The model under review builds one solid part; all positions refer to its coordinate system, in mm. Face numbers are marked on the shaded views. A direction names the side the tool comes from. Coordinates: 2 decimals unless noted, no trailing zeros. Loops run counter-clockwise (first coordinate to the right, second up) from the corner with the lowest first, then second, coordinate; pieces in that order, holes last. Notation, with made-up numbers: M -38,5.25 L 2,5.25 A23 ccw 2,38.25 Z; hole C -34,-21.5 d4. An arc over 180 degrees is marked long. Return JSON: item names as keys, results as strings.
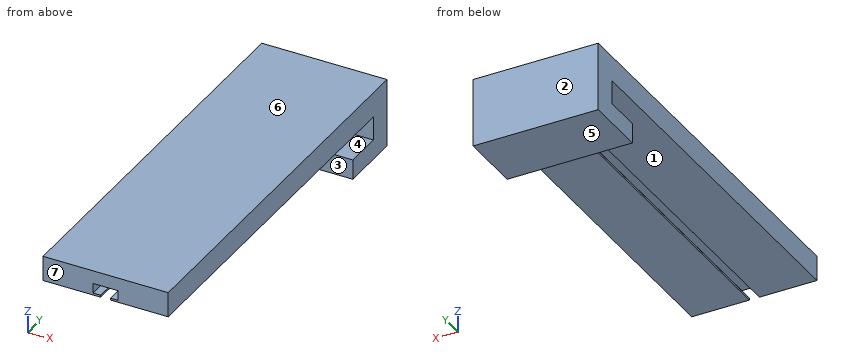
```python
from build123d import *

# Parameters (mm, degrees)
F0_W     = 15.875
F0_H     = 50.8
F1_DEPTH = 3.175
F2_W     = 15.875
F2_H     = 3.175
F3_DEPTH = 5.55625
F4_W     = 15.875
F4_H     = 2.54
F5_DEPTH = 4.7625
F6_W     = 1.27
F6_H     = 0.2512368413
F7_DEPTH = 38.1


with BuildPart() as f1:
    # F0 (on Top) → F1 (new body)
    with BuildSketch(Plane.XY):
        Rectangle(F0_W, F0_H)
    extrude(amount=F1_DEPTH)

    # F2 (on face) → F3 (join)
    with BuildSketch(Plane(origin=(0, 0, 0), x_dir=(1, 0, 0), z_dir=(0, 0, -1))):
        with Locations((0, -23.8125)):
            Rectangle(F2_W, F2_H)
    extrude(amount=F3_DEPTH)

    # F4 (on face) → F5 (join)
    with BuildSketch(Plane.XZ.offset(-22.225)):
        with Locations((0, -4.28625)):
            Rectangle(F4_W, F4_H)
    extrude(amount=F5_DEPTH)

    # F6 (on face) → F7 (cut)
    with BuildSketch(Plane.XZ.offset(25.4)):
        Polygon((0.635, 0.2512368413), (1.5875, 0.2512368413), (1.5875, 1.5212368413), (-1.5875, 1.5212368413), (-1.5875, 0.2512368413), (-0.635, 0.2512368413), align=None)
        with Locations((0, 0.1256184207)):
            Rectangle(F6_W, F6_H)
    extrude(amount=-F7_DEPTH, mode=Mode.SUBTRACT)


solid = f1.part
```
1. Add section C-C on z = -1.75. Give the boundary of the cut face in (x, y) (1 decimal), plus the area to 3 significant figures.
Check values:
{"outline": "M -7.9,22.2 L 7.9,22.2 L 7.9,25.4 L -7.9,25.4 Z", "area": "50.4 mm²"}
2. Add section B-B on x = -3.25. Give the boundary of the cut face in (y, z) (1 decimal).
Check values:
{"outline": "M -25.4,0 L 22.2,0 L 22.2,-3 L 17.5,-3 L 17.5,-5.6 L 25.4,-5.6 L 25.4,3.2 L -25.4,3.2 Z"}
3. To check wall thickness, follow line 1 (X direction, y = -3, z = 1); line 2 (Z direction, x = -6.25, y = 5) (3 decimals); line 3 (Y direction, x = 4, z = -3.5). State the ranges of each line that lie inside material, in increasing order.
Check values:
{"line 1": "-7.94 to -1.59, 1.59 to 7.94", "line 2": "0 to 3.175", "line 3": "17.46 to 25.4"}
4. Insertion check: pin 1 Ø1 at (x, y) = (0.5, -12.5) entering from -Z; pin 2 Ø1.5 at (x, z) = (0.5, -1) entering from -Y (3 decimals); pin 3 Ø0.5 at (x, z) = (0.5, 1) entering from -Y. Each pin has a flat end and moves straight along its axis. Give the tip position at first contact, or say it passes through.
Check values:
{"pin 1": "z = 0", "pin 2": "y = 22.225", "pin 3": "y = 12.7"}
5. Machinability: for the marked faces 1, 2 and 3, which of the approach directions +Z, -Z, +X, -X, +Y, -Y give a long, thin tool a straight path to every point of the face, cutting with its end or side? Answer none if there is none.
Check values:
{"face 1": "+X, -X, -Y", "face 2": "+Z, -Z, +X, -X, +Y", "face 3": "-Z, +X, -X, -Y"}
6. The part is to be moulded in two halves that separate along Z. For the marked faces 4, 5, 6 and 7, say which applies: released by +Z, released by -Z, zero draft, split by the parting line, or undercut.
Check values:
{"face 4": "undercut", "face 5": "released by -Z", "face 6": "released by +Z", "face 7": "zero draft"}
